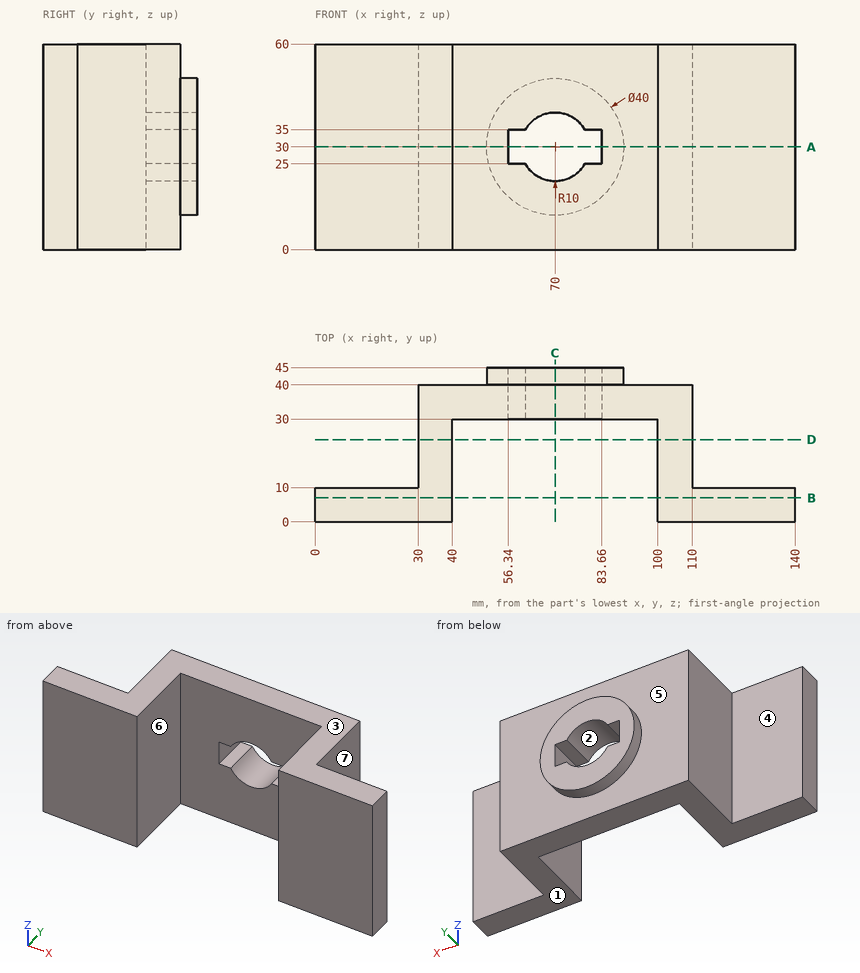
The drawing under review shows one solid part. Ordinate dimensions are in mm from its lowest x, y, z. A direction names the side the tool comes from. Coordinates: 2 decimals unless noted, no trailing zeros. Loops run counter-clockwise (first coordinate to the right, second up) from the corner with the lowest first, then second, coordinate; pieces in that order, holes last. Notation, with made-up numbers: (-8, 49.25) -> (46, 49.25) arc R24 ccw to (46, 71.25) -> close; hole circle Ø5 at (89.25, 13.5). An arc over 180 degrees is marked (long way). Answer as a JSON object with one key per item and string values.
Q1. Clearance check with flat-ended pins moving along their axes: pin 1 Ø1 at (y, z) = (25, 25.5) entering from +X; pin 2 Ø9 at (x, z) = (20, 24.5) entering from +Y; pin 3 Ø6 at (y, z) = (17, 37.5) entering from -X; pin 4 Ø3 at (x, y) = (97.5, 20) entering from +Z. State where each tip first meets the part, or that it passes through.
Answer block:
{"pin 1": "stops at x = 110", "pin 2": "stops at y = 10", "pin 3": "stops at x = 30", "pin 4": "passes through"}
Q2. Take a section at C-C on x = 70. Give the boundary of the cut face in (y, z).
Answer block:
{"outline": "(30, 0) -> (40, 0) -> (40, 10) -> (45, 10) -> (45, 20) -> (30, 20) -> close; (30, 40) -> (45, 40) -> (45, 50) -> (40, 50) -> (40, 60) -> (30, 60) -> close"}
Q3. Take a section at B-B on y = 7. Give the boundary of the cut face in (x, z).
Answer block:
{"outline": "(0, 0) -> (40, 0) -> (40, 60) -> (0, 60) -> close; (100, 0) -> (140, 0) -> (140, 60) -> (100, 60) -> close"}
Q4. Take a section at A-A on z = 30. Give the boundary of the cut face in (x, y).
Answer block:
{"outline": "(0, 0) -> (40, 0) -> (40, 30) -> (56.34, 30) -> (56.34, 45) -> (50, 45) -> (50, 40) -> (30, 40) -> (30, 10) -> (0, 10) -> close; (83.66, 30) -> (100, 30) -> (100, 0) -> (140, 0) -> (140, 10) -> (110, 10) -> (110, 40) -> (90, 40) -> (90, 45) -> (83.66, 45) -> close"}
Q5. Tool access review of the marked faces 5, 6 and 7: name each direction out of +Z, -Z, +X, -X, +Y, -Y from which nothing blocks a thin tool from reaching the whole face with its end or side.
Answer block:
{"face 5": "+Y", "face 6": "+Z, -Z, -Y", "face 7": "+Z, -Z, +X, +Y"}
Q6. Take a section at D-D on y = 24. Give the boundary of the cut face in (x, z), plus the area to 3 significant figures.
Answer block:
{"outline": "(30, 0) -> (40, 0) -> (40, 60) -> (30, 60) -> close; (100, 0) -> (110, 0) -> (110, 60) -> (100, 60) -> close", "area": "1,200 mm^2"}
Q7. To check wall thickness, follow L1, parallel to X at y = 2, z = 9; L2, parallel to Z at x = 58, y = 37; L3, parallel to X at y = 10.5, z = 34.5. State the ranges of each line that lie inside material, in increasing order.
Answer block:
{"L1": "x = 0 to 40, 100 to 140", "L2": "z = 0 to 25, 35 to 60", "L3": "x = 30 to 40, 100 to 110"}
Q8. The part is to be moulded in two halves that separate along Z. For the marked faces 1, 2, 3 and 4, say which applies: +Z half, -Z half, draft (parallel to the pull), parting line (faces both ways), or undercut.
Answer block:
{"face 1": "-Z half", "face 2": "undercut", "face 3": "+Z half", "face 4": "draft"}
